The drawing under review shows one solid part. Ordinate dimensions are in mm from its lowest x, y, z. Round coordinates to 2 decimals unless told otherwise and drop trailing zeros. Order: outer loops, then holes, each group sorted by start corner. A loop starts at its lowest first (then second) coordinate and runs counter-clockwise, first axis right, second up. Notation, with made-up numbers: M 57,49 L 71,49 A6 cw 71,56 Z; hole C -9,67 d3. An arc over 180 degrees is marked long. Answer as a JSON object with one key per item and string values. Group by question number.
1. Add section B-B on z = 7.5. State the section outline as (x, y) points, and give its area (3 significant figures).
2. Add section D-D on y = 6.75. State the section outline as (x, z) points (3 decimals).
3. To check wall thickness, follow probe 1 along Z at (x, y) = (9.5, 2.5); probe 2 along Z at (x, y) = (10.25, 9). State the ranges of each line that lie inside material, in increasing order. Write a range as [from, to].
4. Add section C-C on z = 5.25. State the section outline as (x, y) points, and give its area (3 significant figures).
5. Add section A-A on x = 9. State the section outline as (y, z) points.
6. Mouldability with a two-part tool opening along Z and no side actions: class the marked faces 1, 2 and 3 as released by +Z, released by -Z, zero draft, split by the parting line, or undercut.
7. Clearance check with a flat-ended pin moving along its axis: P1, Ø1, axis at x = 5, y = 2, coming from the +Z side. State where the tip first meets the part, or that it passes through.
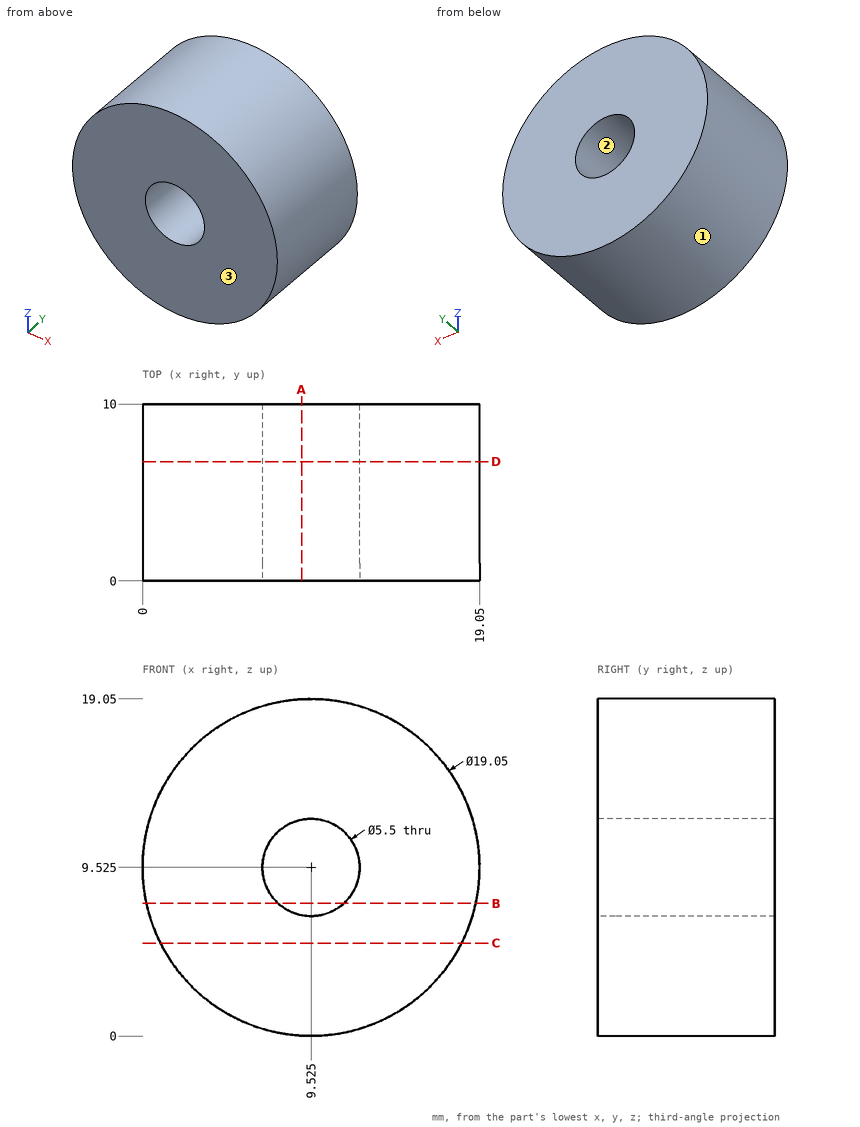
Recorded:
{
 "1": {"outline": "M 0.22,0 L 7.66,0 L 7.66,10 L 0.22,10 Z; M 11.39,0 L 18.83,0 L 18.83,10 L 11.39,10 Z", "area": "149 mm²"},
 "2": {"outline": "C 9.525,9.525 d19.05; hole C 9.525,9.525 d5.5"},
 "3": {"probe 1": "z = [0, 6.78], [12.27, 19.05]", "probe 2": "z = [0.03, 6.87], [12.18, 19.02]"},
 "4": {"outline": "M 1.01,0 L 18.04,0 L 18.04,10 L 1.01,10 Z", "area": "170 mm²"},
 "5": {"outline": "M 0,0.01 L 10,0.01 L 10,6.83 L 0,6.83 Z; M 0,12.22 L 10,12.22 L 10,19.04 L 0,19.04 Z"},
 "6": {"face 1": "split by the parting line", "face 2": "undercut", "face 3": "zero draft"},
 "7": {"P1": "stops at z = 18.16"}
}
